CAD build for the part. Positions are in the model's coordinates, mm. A direction names the side the tool comes from. Give positions to 0.01 mm unless a question says otherwise; leave off trailing zeros. Loops run counter-clockwise (first coordinate to the right, second up) from the corner with the lowest first, then second, coordinate; pieces in that order, holes last. Notation, with made-up numbers: (51, 1) - (63, 1) arc R30 ccw to (63, 39) - close; hole circle Ø10 at (0, 77). An arc over 180 degrees is marked (long way). Return JSON: item names as keys, results as strings.
from build123d import *

# Parameters (mm, degrees)
SKETCH_1_W      = 67
SKETCH_1_H      = 115
SKETCH_1_R      = 1.05
EXTRUDE_1_DEPTH = 2


with BuildPart() as part:
    # 草图1 → 凸台-拉伸1 (new body)
    with BuildSketch(Plane(origin=(0, 0, 0), x_dir=(1, 0, 0), z_dir=(0, 1, 0))):
        with Locations((33.5, -57.5)):
            Rectangle(SKETCH_1_W, SKETCH_1_H)
        with Locations(Location((2, -113, 0), (0, 0, 270))):
            Circle(SKETCH_1_R, mode=Mode.SUBTRACT)
        with Locations(Location((65, -113, 0), (0, 0, 270))):
            Circle(SKETCH_1_R, mode=Mode.SUBTRACT)
        Polygon((6.5, -103.5), (6.5, -11.5), (60.5, -11.5), (60.5, -77), (62.5, -77), (62.5, -95), (60.5, -95), (60.5, -103.5), align=None, mode=Mode.SUBTRACT)
        with Locations(Location((2, -2, 0), (0, 0, 270))):
            Circle(SKETCH_1_R, mode=Mode.SUBTRACT)
        with Locations(Location((65, -2, 0), (0, 0, 270))):
            Circle(SKETCH_1_R, mode=Mode.SUBTRACT)
    extrude(amount=EXTRUDE_1_DEPTH)


solid = part.part
1. Cut at C-C, the plane z = 83.5. Write the cut outline in (x, y).
Values follow:
{"outline": "(0, 0) - (6.5, 0) - (6.5, 2) - (0, 2) - close; (62.5, 0) - (67, 0) - (67, 2) - (62.5, 2) - close"}
2. Drill centre lines: probe 1 along X at (y, z) = (1.55, 2); probe 2 along Z at (x, y) = (7, 0.9); probe 3 along X at (y, z) = (1.65, 78). Where is each one in solid material? Low to high.
Values follow:
{"probe 1": "x = 0 to 0.95, 3.05 to 63.95, 66.05 to 67", "probe 2": "z = 0 to 11.5, 103.5 to 115", "probe 3": "x = 0 to 6.5, 62.5 to 67"}
3. Drop a flat-ended pin along its axis: P1, Ø1.7, axis at x = 65, z = 2, coming from the -Y side. Give the stop position or say it passes through.
Values follow:
{"P1": "passes through"}
4. Cut at A-A, the plane y = 0.9. Write the cut outline in (x, z).
Values follow:
{"outline": "(0, 0) - (67, 0) - (67, 115) - (0, 115) - close; hole circle Ø2.1 at (2, 2); hole circle Ø2.1 at (2, 113); hole (6.5, 11.5) - (60.5, 11.5) - (60.5, 77) - (62.5, 77) - (62.5, 95) - (60.5, 95) - (60.5, 103.5) - (6.5, 103.5) - close; hole circle Ø2.1 at (65, 2); hole circle Ø2.1 at (65, 113)"}
5. Cut at B-B, the plane z = 99. Write the cut outline in (x, y), plus the area to 3 significant figures.
Values follow:
{"outline": "(0, 0) - (6.5, 0) - (6.5, 2) - (0, 2) - close; (60.5, 0) - (67, 0) - (67, 2) - (60.5, 2) - close", "area": "26.0 mm²"}
6. Which spindle directions (+Z, -Z, +X, -X, +Y, -Y) get a long thin tool onto all of the face, cutting with end or side? Do faces 5 (the face through (3, 2, 57)), 6 (the face through (62.5, 1, 86)). Say none if no direction does.
Values follow:
{"face 5": "+Z, -Z, +X, -X, +Y", "face 6": "+Y, -Y"}
7. Pull direction Z, two halves, no side cores. Call faces 1 (the face through (3, 0, 57)), 2 (the face through (65.05, 0.99, 111.95)), 3 (the face through (61, 1, 77)), 4 (the face through (33, 1, 0)): +Z half, -Z half, draft (parallel to the pull), parting line (faces both ways), or undercut.
Values follow:
{"face 1": "draft", "face 2": "undercut", "face 3": "undercut", "face 4": "-Z half"}
